from build123d import *

# Parameters (mm, degrees)
BOSS_EXTRUDE1_DEPTH                                 = 60
CUT_EXTRUDE1_DEPTH                                  = 105.043260233
CBORE_FOR_M3_HEX_SOCKET_HEAD_CAP_SCREW1_D           = 3.4
CBORE_FOR_M3_HEX_SOCKET_HEAD_CAP_SCREW1_CBORE_D     = 6.5
CBORE_FOR_M3_HEX_SOCKET_HEAD_CAP_SCREW1_CBORE_DEPTH = 3
CUT_EXTRUDE5_REACH                                  = 106.043
CUT_EXTRUDE6_DEPTH                                  = 3
M5_TAPPED_HOLE1_D                                   = 4.2
M4_TAPPED_HOLE1_D                                   = 3.3
M4_TAPPED_HOLE1_DEPTH                               = 6
M4_TAPPED_HOLE1_CSINK_D                             = 4.5
M4_TAPPED_HOLE1_CSINK_ANGLE                         = 90
M5_TAPPED_HOLE2_D                                   = 4.2
M5_TAPPED_HOLE2_DEPTH                               = 6
M5_TAPPED_HOLE2_CSINK_D                             = 5.05
M5_TAPPED_HOLE2_CSINK_ANGLE                         = 90


with BuildPart() as part:
    # Sketch1 → Boss-Extrude1 (new body)
    with BuildSketch(Plane.XY):
        Polygon((0, 0), (6, 0), (6, 34), (69, 34), (69, 20), (75, 20), (75, 40), (0, 40), align=None)
    extrude(amount=BOSS_EXTRUDE1_DEPTH)

    # Sketch2 → Cut-Extrude1 (cut, through all)
    with BuildSketch(Plane(origin=(0, 40, 0), x_dir=(1, 0, 0), z_dir=(0, 1, 0))):
        with BuildLine():
            Line((40, -18.5), (50, -18.5))
            ThreePointArc((50, -18.5), (61.5, -30), (50, -41.5))
            Line((50, -41.5), (40, -41.5))
            ThreePointArc((40, -41.5), (28.5, -30), (40, -18.5))
        make_face()
    extrude(amount=-CUT_EXTRUDE1_DEPTH, mode=Mode.SUBTRACT)

    # CBORE for M3 Hex Socket Head Cap Screw1 (through all)
    with Locations(Plane(origin=(0, 40, 0), x_dir=(-1, 0, 0), z_dir=(0, 1, 0))):
        with Locations((-24.5, 45.5), (-55.5, 45.5), (-24.5, 14.5), (-55.5, 14.5)):
            CounterBoreHole(CBORE_FOR_M3_HEX_SOCKET_HEAD_CAP_SCREW1_D / 2, CBORE_FOR_M3_HEX_SOCKET_HEAD_CAP_SCREW1_CBORE_D / 2, CBORE_FOR_M3_HEX_SOCKET_HEAD_CAP_SCREW1_CBORE_DEPTH)

    # Sketch24 → Cut-Extrude5 (cut, up to next)
    with BuildSketch(Plane(origin=(0, 40, 0), x_dir=(1, 0, 0), z_dir=(0, 1, 0)), mode=Mode.PRIVATE) as cut_extrude5_sk1:
        with BuildLine():
            Line((24.5, -12.8), (34.5, -12.8))
            ThreePointArc((34.5, -12.8), (36.2, -14.5), (34.5, -16.2))
            Line((34.5, -16.2), (24.5, -16.2))
            ThreePointArc((24.5, -16.2), (22.8, -14.5), (24.5, -12.8))
        make_face()
    cut_extrude5_tool1 = extrude(cut_extrude5_sk1.sketch, amount=-CUT_EXTRUDE5_REACH, mode=Mode.PRIVATE) & part.part
    # Sketch24 → Cut-Extrude5 (cut, up to next)
    with BuildSketch(Plane(origin=(0, 40, 0), x_dir=(1, 0, 0), z_dir=(0, 1, 0)), mode=Mode.PRIVATE) as cut_extrude5_sk2:
        with BuildLine():
            Line((55.5, -12.8), (65.5, -12.8))
            ThreePointArc((65.5, -12.8), (67.2, -14.5), (65.5, -16.2))
            Line((65.5, -16.2), (55.5, -16.2))
            ThreePointArc((55.5, -16.2), (53.8, -14.5), (55.5, -12.8))
        make_face()
    cut_extrude5_tool2 = extrude(cut_extrude5_sk2.sketch, amount=-CUT_EXTRUDE5_REACH, mode=Mode.PRIVATE) & part.part
    # Sketch24 → Cut-Extrude5 (cut, up to next)
    with BuildSketch(Plane(origin=(0, 40, 0), x_dir=(1, 0, 0), z_dir=(0, 1, 0)), mode=Mode.PRIVATE) as cut_extrude5_sk3:
        with BuildLine():
            Line((24.5, -43.8), (34.5, -43.8))
            ThreePointArc((34.5, -43.8), (36.2, -45.5), (34.5, -47.2))
            Line((34.5, -47.2), (24.5, -47.2))
            ThreePointArc((24.5, -47.2), (22.8, -45.5), (24.5, -43.8))
        make_face()
    cut_extrude5_tool3 = extrude(cut_extrude5_sk3.sketch, amount=-CUT_EXTRUDE5_REACH, mode=Mode.PRIVATE) & part.part
    # Sketch24 → Cut-Extrude5 (cut, up to next)
    with BuildSketch(Plane(origin=(0, 40, 0), x_dir=(1, 0, 0), z_dir=(0, 1, 0)), mode=Mode.PRIVATE) as cut_extrude5_sk4:
        with BuildLine():
            Line((55.5, -43.8), (65.5, -43.8))
            ThreePointArc((65.5, -43.8), (67.2, -45.5), (65.5, -47.2))
            Line((65.5, -47.2), (55.5, -47.2))
            ThreePointArc((55.5, -47.2), (53.8, -45.5), (55.5, -43.8))
        make_face()
    cut_extrude5_tool4 = extrude(cut_extrude5_sk4.sketch, amount=-CUT_EXTRUDE5_REACH, mode=Mode.PRIVATE) & part.part
    add(cut_extrude5_tool1.solids().sort_by_distance((29.5, 40, 14.5))[0], mode=Mode.SUBTRACT)
    add(cut_extrude5_tool2.solids().sort_by_distance((60.5, 40, 14.5))[0], mode=Mode.SUBTRACT)
    add(cut_extrude5_tool3.solids().sort_by_distance((29.5, 40, 45.5))[0], mode=Mode.SUBTRACT)
    add(cut_extrude5_tool4.solids().sort_by_distance((60.5, 40, 45.5))[0], mode=Mode.SUBTRACT)

    # Sketch25 → Cut-Extrude6 (cut)
    with BuildSketch(Plane(origin=(0, 40, 0), x_dir=(1, 0, 0), z_dir=(0, 1, 0))):
        with BuildLine():
            Line((24.5, -11.25), (34.5, -11.25))
            ThreePointArc((34.5, -11.25), (37.75, -14.5), (34.5, -17.75))
            Line((34.5, -17.75), (24.5, -17.75))
            ThreePointArc((24.5, -17.75), (21.25, -14.5), (24.5, -11.25))
        make_face()
        with BuildLine():
            Line((55.499988687, -11.3096476), (65.499988687, -11.3096476))
            ThreePointArc((65.499988687, -11.3096476), (68.749988687, -14.5596476), (65.499988687, -17.8096476))
            Line((65.499988687, -17.8096476), (55.499988687, -17.8096476))
            ThreePointArc((55.499988687, -17.8096476), (52.249988687, -14.5596476), (55.499988687, -11.3096476))
        make_face()
        with BuildLine():
            Line((24.5, -42.25), (34.5, -42.25))
            ThreePointArc((34.5, -42.25), (37.75, -45.5), (34.5, -48.75))
            Line((34.5, -48.75), (24.5, -48.75))
            ThreePointArc((24.5, -48.75), (21.25, -45.5), (24.5, -42.25))
        make_face()
        with BuildLine():
            Line((55.499988687, -42.3096476), (65.499988687, -42.3096476))
            ThreePointArc((65.499988687, -42.3096476), (68.749988687, -45.5596476), (65.499988687, -48.8096476))
            Line((65.499988687, -48.8096476), (55.499988687, -48.8096476))
            ThreePointArc((55.499988687, -48.8096476), (52.249988687, -45.5596476), (55.499988687, -42.3096476))
        make_face()
    extrude(amount=-CUT_EXTRUDE6_DEPTH, mode=Mode.SUBTRACT)

    # M5 Tapped Hole1 (through all)
    with Locations(Plane(origin=(0, 40, 0), x_dir=(-1, 0, 0), z_dir=(0, 1, 0))):
        with Locations((-44, 12), (-44, 48)):
            Hole(M5_TAPPED_HOLE1_D / 2)

    # M4 Tapped Hole1
    with Locations(Plane.ZY):
        with Locations((11, 20), (49, 20)):
            CounterSinkHole(M4_TAPPED_HOLE1_D / 2, M4_TAPPED_HOLE1_CSINK_D / 2, depth=M4_TAPPED_HOLE1_DEPTH, counter_sink_angle=M4_TAPPED_HOLE1_CSINK_ANGLE)

    # M5 Tapped Hole2
    with Locations(Plane(origin=(75, 0, 0), x_dir=(0, 0, -1), z_dir=(1, 0, 0))):
        with Locations((-30, 30)):
            CounterSinkHole(M5_TAPPED_HOLE2_D / 2, M5_TAPPED_HOLE2_CSINK_D / 2, depth=M5_TAPPED_HOLE2_DEPTH, counter_sink_angle=M5_TAPPED_HOLE2_CSINK_ANGLE)


solid = part.part
Here's how the part is built. I have some questions about the finished solid (model axes, mm). A direction names the side the tool comes from. Coordinates: 2 decimals unless noted, no trailing zeros. Loops run counter-clockwise (first coordinate to the right, second up) from the corner with the lowest first, then second, coordinate; pieces in that order, holes last.
1. Imagine slicing it at B-B, the plane z = 35. Please give me the cut outline in (x, y), and give its area (3 significant figures).
2. If we mould it in two halves opening along X, with no side actions, what happens to faces 4 (the flat face through (72, 20, 30)), 5 (the cylindrical face through (37.75, 38.52, 14.43)), 6 (the flat face through (0, 20, 30))? For each: pulls with the +X half, pulls with the -X half, needs draft (parallel to the pull), parting line crosses it, or undercut.
3. Imagine slicing it at C-C, the plane x = 9. Please give me the cut outline in (y, z).
4. Imagine slicing it at D-D, the plane y = 10.5. Please give me the cut outline in (x, z), and give its area (3 significant figures).
5. For P1, Ø5, axis at x = 46, y = 36.5, coming from the -Z side; P2, Ø2.5, axis at y = 30, z = 30, coming from the +X side; P3, Ø2, axis at y = 20, z = 49, coming from the -X side; P4, Ø3.5, axis at x = 63, z = 13.5, coming from the +Y side, each with a flat end and sliding along its axis, tell me the tip position at first contact or that it passes through.
6. I need wall thicknesses on L1, parallel to Z at x = 3, y = 20; L2, parallel to Y at x = 2.1, z = 49; L3, parallel to Y at x = 72, z = 30. Which ranges of each line are inside material? Lowest first, please.
7. Imagine slicing it at A-A, the plane z = 54. Please give me the cut outline in (x, y).
8. For faces 1 (the flat face through (32, 36, 60)), 2 (the flat face through (29, 39, 42.25)), 3 (the flat face through (30, 36, 16.2)), which set-ups out of +Z, -Z, +X, -X, +Y, -Y let a thin tool reach every point of the face, with its end or its side?
Taken from the geometry:
1. outline: (0, 0) - (6, 0) - (6, 34) - (29.64, 34) - (29.64, 40) - (0, 40) - close; (60.36, 34) - (69, 34) - (69, 20) - (75, 20) - (75, 40) - (60.36, 40) - close
1. area: 554 mm2
2. face 4: needs draft
2. face 5: undercut
2. face 6: pulls with the -X half
3. outline: (34, 0) - (40, 0) - (40, 60) - (34, 60) - close
4. outline: (0, 0) - (6, 0) - (6, 60) - (0, 60) - close
4. area: 360 mm2
5. P1: stops at z = 0
5. P2: stops at x = 6
5. P3: stops at x = 69
5. P4: stops at y = 37
6. L1: z = 0 to 9.35, 12.65 to 47.35, 50.65 to 60
6. L2: y = 0 to 18.35, 21.65 to 40
6. L3: y = 20 to 27.9, 32.1 to 40
7. outline: (0, 0) - (6, 0) - (6, 34) - (69, 34) - (69, 20) - (75, 20) - (75, 40) - (0, 40) - close
8. face 1: +Z, +X, -X, +Y, -Y
8. face 2: +Y
8. face 3: +Y, -Y
